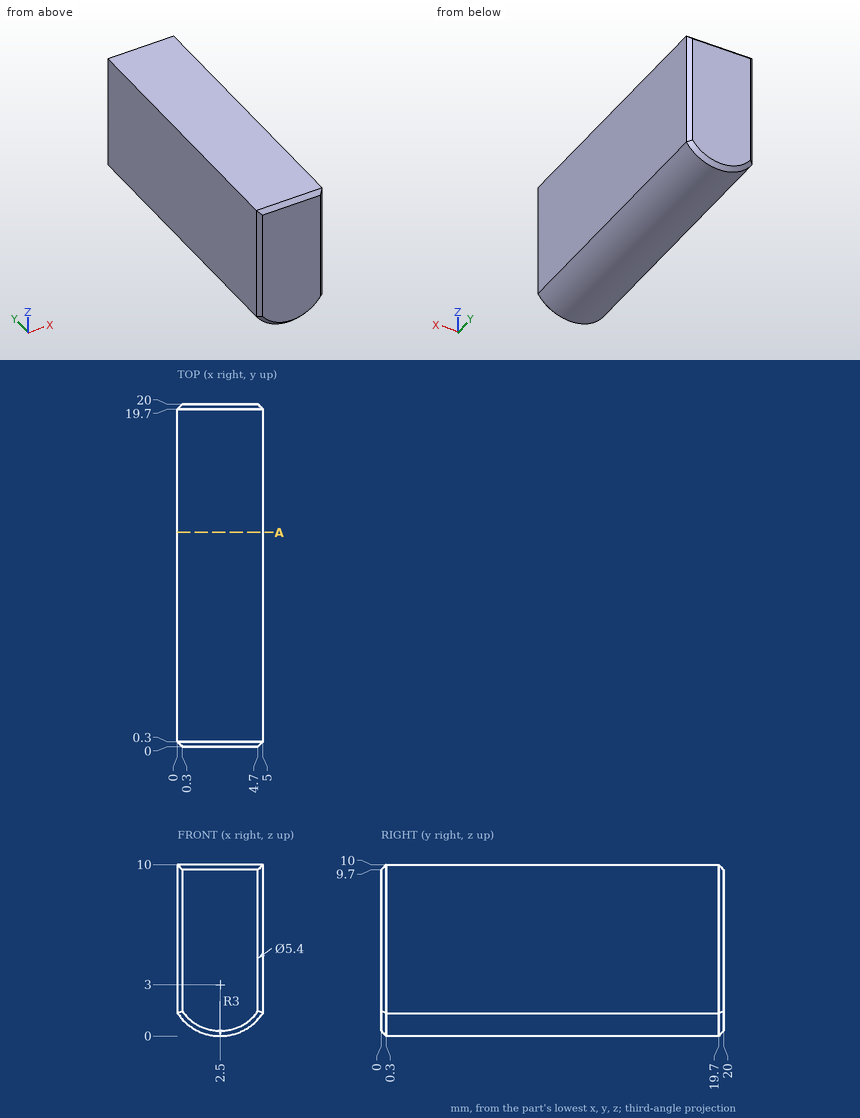
Geometry: see drawing. Coordinates: mm, zero at the bounding-box minimum. Give positions to 0.01 mm unless a question says otherwise; leave off trailing zeros. Loops run counter-clockwise (first coordinate to the right, second up) from the corner with the lowest first, then second, coordinate; pieces in that order, holes last. Notation, with made-up numbers: (45, 52) - (87, 52) arc R7 cw to (87, 64) - close; hole circle Ø4 at (81.5, -3.5). An arc over 180 degrees is marked (long way). Use CSV: the item, a comma, the result in double quotes.
1) Line query: line 1 (Z direction, x = 2.6, y = 5.75); line 2 (Z direction, x = 3.8, y = 19.25); line 3 (X direction, y = 13.5, z = 0.75). Output: solid intervals per line, ascending.
Worked out:
line 1,"z = 0 to 10"
line 2,"z = 0.3 to 10"
line 3,"x = 0.52 to 4.48"
2) Pin query (flat end, axial travel): P1, Ø1, axis at x = 4, y = 16.5, coming from the -Z side. Return the tip coordinate at first contact, or that it passes through.
Worked out:
P1,"stops at z = 0.17"
3) Cut plane A-A (y = 12.5). Output: boundary loops of the cut face in (x, z), and give its area (3 significant figures).
Worked out:
outline,"(0, 1.34) arc R3 ccw to (5, 1.34) - (5, 10) - (0, 10) - close"
area,"48.0 mm^2"
